For this review, take the finished solid that the model builds, in its own axes (mm). Coordinates: 2 decimals unless noted, no trailing zeros. Loops run counter-clockwise (first coordinate to the right, second up) from the corner with the lowest first, then second, coordinate; pieces in that order, holes last. Notation, with made-up numbers: (54, -12) -> (60, -12) arc R15 ccw to (60, 15) -> close; hole circle Ø1 at (17, -32). An arc over 180 degrees is marked (long way). One line per item, written item: value.
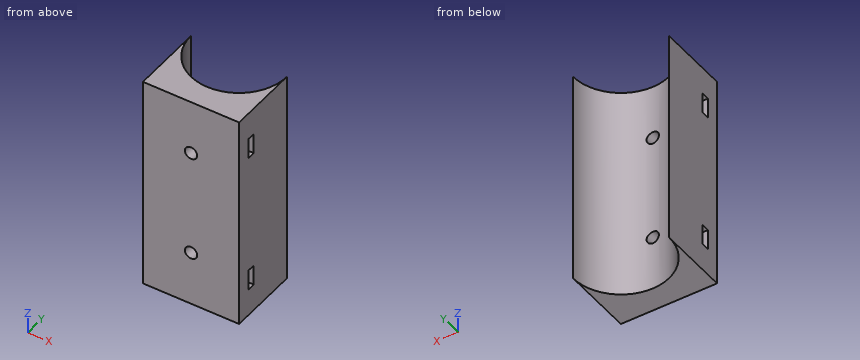
from build123d import *

# Parameters (mm, degrees)
BOSS_EXTRU_1_DEPTH      = 79.1
D_GAGEMENT_M41_D        = 4.5
D_GAGEMENT_M41_DEPTH    = 10
D_GAGEMENT_M41_TIP      = 1.351936393
ESQUISSE7_W             = 7.5
ESQUISSE7_H             = 3
BOSS_EXTRU_3_DEPTH      = 35
ESQUISSE7_2_W           = 7.5
ESQUISSE7_2_H           = 3
ENL_V_MAT_EXTRU_5_DEPTH = 35


with BuildPart() as part:
    # Esquisse1 → Boss.-Extru.1 (new body)
    with BuildSketch(Plane.XY.offset(1608.553140947)):
        with BuildLine():
            Line((0, 0), (35, 0))
            Line((35, 0), (35, 26.25))
            ThreePointArc((35, 26.25), (17.5, 8.75), (0, 26.25))
            Line((0, 26.25), (0, 0))
        make_face()
    extrude(amount=BOSS_EXTRU_1_DEPTH)

    # Dégagement M41
    with Locations(Plane(origin=(17.499999998, 8.75, 1628.553140947), x_dir=(1.0, -1.24e-10, 0), z_dir=(1.24e-10, 1.0, 0))):
        with Locations((0, 0), (2e-09, -39.1)):
            Hole(D_GAGEMENT_M41_D / 2, depth=D_GAGEMENT_M41_DEPTH)
            with Locations((0, 0, -(D_GAGEMENT_M41_DEPTH + D_GAGEMENT_M41_TIP / 2))):  # 118° drill point
                Cone(0, D_GAGEMENT_M41_D / 2, D_GAGEMENT_M41_TIP, mode=Mode.SUBTRACT)

    # Esquisse7 → Boss.-Extru.3 (add)
    with BuildSketch(Plane(origin=(35, 0, 0), x_dir=(0, 0, -1), z_dir=(1, 0, 0))):
        with Locations((-1673.903140947, 6.5)):
            Rectangle(ESQUISSE7_W, ESQUISSE7_H)
        with Locations((-1622.303140947, 6.5)):
            Rectangle(ESQUISSE7_W, ESQUISSE7_H)
    extrude(amount=-BOSS_EXTRU_3_DEPTH)

    # Esquisse7<2> → Enlèv. mat.-Extru.5 (cut)
    with BuildSketch(Plane(origin=(35, 0, 0), x_dir=(0, 0, -1), z_dir=(1, 0, 0))):
        with Locations((-1673.903140947, 6.5)):
            Rectangle(ESQUISSE7_2_W, ESQUISSE7_2_H)
        with Locations((-1622.303140947, 6.5)):
            Rectangle(ESQUISSE7_2_W, ESQUISSE7_2_H)
    extrude(amount=-ENL_V_MAT_EXTRU_5_DEPTH, mode=Mode.SUBTRACT)


solid = part.part
1. Take a section at D-D, the plane y = 11.5. Give the boundary of the cut face in (x, z).
Return value:
outline: (0, 1608.55) -> (8.08, 1608.55) -> (8.08, 1687.65) -> (0, 1687.65) -> close; (26.92, 1608.55) -> (35, 1608.55) -> (35, 1687.65) -> (26.92, 1687.65) -> close
2. Take a section at B-B, the plane y = 21.25. Give the boundary of the cut face in (x, z).
Return value:
outline: (0, 1608.55) -> (0.73, 1608.55) -> (0.73, 1687.65) -> (0, 1687.65) -> close; (34.27, 1608.55) -> (35, 1608.55) -> (35, 1687.65) -> (34.27, 1687.65) -> close
3. Take a section at A-A, the plane x = 17.5. Give the boundary of the cut face in (y, z), and give its area (3 significant figures).
Return value:
outline: (0, 1608.55) -> (8.75, 1608.55) -> (8.75, 1626.3) -> (0, 1626.3) -> close; (0, 1630.8) -> (8.75, 1630.8) -> (8.75, 1665.4) -> (0, 1665.4) -> close; (0, 1669.9) -> (8.75, 1669.9) -> (8.75, 1687.65) -> (0, 1687.65) -> close; hole (5, 1618.55) -> (8, 1618.55) -> (8, 1626.05) -> (5, 1626.05) -> close; hole (5, 1670.15) -> (8, 1670.15) -> (8, 1677.65) -> (5, 1677.65) -> close
area: 568 mm2
4. Insertion check: pin 1 Ø8 at (x, z) = (18, 1621) entering from +Y; pin 2 Ø6 at (x, z) = (18, 1674) entering from +Y. Each pin has a flat end and moves straight along its axis. Give the tip position at first contact, or say it passes through.
Return value:
pin 1: stops at y = 9.34
pin 2: stops at y = 9.1
5. To check wall thickness, follow probe 1 along Z at (x, y) = (17.5, 2); probe 2 along Z at (x, y) = (17.5, 6); probe 3 along Z at (x, y) = (19, 8.5). State the ranges of each line that lie inside material, in increasing order. Write a range as from..to.
Return value:
probe 1: z = 1608.55..1626.3, 1630.8..1665.4, 1669.9..1687.65
probe 2: z = 1608.55..1618.55, 1626.05..1626.3, 1630.8..1665.4, 1669.9..1670.15, 1677.65..1687.65
probe 3: z = 1608.55..1626.88, 1630.23..1665.98, 1669.33..1687.65
6. Take a section at C-C, the plane x = 23. Give the boundary of the cut face in (y, z), and give its area (3 significant figures).
Return value:
outline: (0, 1608.55) -> (9.64, 1608.55) -> (9.64, 1687.65) -> (0, 1687.65) -> close; hole (5, 1618.55) -> (8, 1618.55) -> (8, 1626.05) -> (5, 1626.05) -> close; hole (5, 1670.15) -> (8, 1670.15) -> (8, 1677.65) -> (5, 1677.65) -> close
area: 717 mm2
